Design review of the part built by this model. Coordinates are the model's own, in mm. A direction names the side the tool comes from. Round coordinates to 2 decimals unless told otherwise and drop trailing zeros. Order: outer loops, then holes, each group sorted by start corner. A loop starts at its lowest first (then second) coordinate and runs counter-clockwise, first axis right, second up.
from build123d import *

# Parameters (mm, degrees)
SKETCH1_W                       = 30
SKETCH1_H                       = 194.2
SKETCH1_H_2                     = 27
SKETCH1_H_3                     = 261.4
EXTRUDE1_DEPTH                  = 15
FILLET1_R                       = 10
EXTRUDE2_DEPTH                  = 10
SKETCH3_W                       = 80
SKETCH3_H                       = 25
EXTRUDE3_DEPTH                  = 30
SKETCH5_W                       = 70
SKETCH5_H                       = 20
EXTRUDE4_DEPTH                  = 24
FILLET2_R                       = 10
EXTRUDE5_REACH                  = 432.349
SKETCH6_R                       = 4.029178008
SKETCH7_W                       = 30
SKETCH7_H                       = 263.372286267
EXTRUDE6_DEPTH                  = 427.91910061
EXTRUDE7_DEPTH                  = 100
SKETCH9_W                       = 30
SKETCH9_H                       = 136.58118173
EXTRUDE8_DEPTH                  = 10
F_1_4_0_25_DIAMETER_HOLE1_D     = 6.35
F_1_4_0_25_DIAMETER_HOLE1_DEPTH = 10
F_1_4_0_25_DIAMETER_HOLE1_TIP   = 1.907732465
EXTRUDE12_DEPTH                 = 20
EXTRUDE12_DEPTH_BACK            = 30
SKETCH11_W                      = 15
SKETCH11_H                      = 6.378618897


with BuildPart() as part:
    # Sketch1 → Extrude1 (new body)
    with BuildSketch(Plane.XY):
        with Locations((15, 322.665015772)):
            Rectangle(SKETCH1_W, SKETCH1_H)
        with BuildLine():
            Line((30, 225.565015772), (30, 198.565015772))
            Line((30, 198.565015772), (50, 198.565015772))
            ThreePointArc((50, 198.565015772), (63.5, 212.065015772), (50, 225.565015772))
            Line((50, 225.565015772), (30, 225.565015772))
        make_face()
        with Locations((15, 212.065015772)):
            Rectangle(SKETCH1_W, SKETCH1_H_2)
        with BuildLine():
            Line((-20, 198.565015772), (0, 198.565015772))
            Line((0, 198.565015772), (0, 225.565015772))
            Line((0, 225.565015772), (-20, 225.565015772))
            ThreePointArc((-20, 225.565015772), (-33.5, 212.065015772), (-20, 198.565015772))
        make_face()
        with Locations((15, 67.865015772)):
            Rectangle(SKETCH1_W, SKETCH1_H_3)
    extrude(amount=EXTRUDE1_DEPTH)

    # Fillet1
    fillet1_edges = [part.edges().sort_by_distance(p)[0] for p in [
        (0, 419.765015772, 7.5),
        (30, 419.765015772, 7.5),
        (30, -62.834984228, 7.5),
        (0, -62.834984228, 7.5),
    ]]
    fillet(fillet1_edges, radius=FILLET1_R)

    # Sketch2 → Extrude2 (cut)
    with BuildSketch(Plane(origin=(0, 0, 0), x_dir=(-1, 0, 0), z_dir=(0, 0, -1))):
        with BuildLine():
            Line((-50, 225.565015772), (-30, 225.565015772))
            Line((-30, 225.565015772), (-30, 198.565015772))
            Line((-30, 198.565015772), (-50, 198.565015772))
            ThreePointArc((-50, 198.565015772), (-63.5, 212.065015772), (-50, 225.565015772))
        make_face()
        with BuildLine():
            Line((0, 198.565015772), (20, 198.565015772))
            ThreePointArc((20, 198.565015772), (33.5, 212.065015772), (20, 225.565015772))
            Line((20, 225.565015772), (0, 225.565015772))
            Line((0, 225.565015772), (0, 198.565015772))
        make_face()
    extrude(amount=-EXTRUDE2_DEPTH, mode=Mode.SUBTRACT)

    # Sketch3 → Extrude3 (add)
    with BuildSketch(Plane.XY.offset(15)):
        with Locations((15, 407.265015772)):
            Rectangle(SKETCH3_W, SKETCH3_H)
    extrude(amount=EXTRUDE3_DEPTH)

    # Sketch5 → Extrude4 (cut)
    with BuildSketch(Plane.XY.offset(45)):
        with Locations((15, 409.765015772)):
            Rectangle(SKETCH5_W, SKETCH5_H)
    extrude(amount=-EXTRUDE4_DEPTH, mode=Mode.SUBTRACT)

    # Fillet2
    fillet2_edges = [part.edges().sort_by_distance(p)[0] for p in [
        (52.5, 419.765015772, 45),
        (-22.5, 419.765015772, 45),
    ]]
    fillet(fillet2_edges, radius=FILLET2_R)

    # Sketch6 → Extrude5 (add, up to next)
    with BuildSketch(Plane.ZY.offset(-50), mode=Mode.PRIVATE) as extrude5_sk1:
        with Locations(Location((35, 413.847695375, 0), (0, 0, 180))):
            Circle(SKETCH6_R)
    extrude5_tool1 = extrude(extrude5_sk1.sketch, amount=EXTRUDE5_REACH, mode=Mode.PRIVATE) - part.part
    add(extrude5_tool1.solids().sort_by_distance((50, 413.847695, 35))[0])

    # Sketch7 → Extrude6 (cut, through all)
    with BuildSketch(Plane(origin=(0, 0, 0), x_dir=(-1, 0, 0), z_dir=(0, 0, -1))):
        with Locations((-15, 66.878872639)):
            Rectangle(SKETCH7_W, SKETCH7_H)
    extrude(amount=-EXTRUDE6_DEPTH, mode=Mode.SUBTRACT)

    # Sketch8 → Extrude7 (add)
    with BuildSketch(Plane(origin=(0, 0, 0), x_dir=(-1, 0, 0), z_dir=(0, 0, -1))):
        Polygon((-30, 198.565015772), (0, 198.565015772), (0, 225.565015772), (-5, 225.565015772), (-5, 203.565015772), (-25, 203.565015772), (-25, 225.565015772), (-30, 225.565015772), align=None)
    extrude(amount=EXTRUDE7_DEPTH)

    # Sketch9 → Extrude8 (add)
    with BuildSketch(Plane(origin=(0, 0, -100), x_dir=(-1, 0, 0), z_dir=(0, 0, -1))):
        with Locations((-15, 157.274424907)):
            Rectangle(SKETCH9_W, SKETCH9_H)
    extrude(amount=EXTRUDE8_DEPTH)

    # 1/4 (0.25) Diameter Hole1
    with Locations(Plane(origin=(-20, 212.065015772, 10), x_dir=(-1, 0, 0), z_dir=(0, 0, -1))):
        with Locations((0, 0), (-70, 0)):
            Hole(F_1_4_0_25_DIAMETER_HOLE1_D / 2, depth=F_1_4_0_25_DIAMETER_HOLE1_DEPTH)
            with Locations((0, 0, -(F_1_4_0_25_DIAMETER_HOLE1_DEPTH + F_1_4_0_25_DIAMETER_HOLE1_TIP / 2))):  # 118° drill point
                Cone(0, F_1_4_0_25_DIAMETER_HOLE1_D / 2, F_1_4_0_25_DIAMETER_HOLE1_TIP, mode=Mode.SUBTRACT)

    # Sketch11 → Extrude12 (add, two sides: drawn at the far end of the back side and taken through both)
    with BuildSketch(Plane.XZ.offset(-88.983834042).offset(-EXTRUDE12_DEPTH_BACK)):
        Polygon((0, -116.378618897), (-22.784065685, -134.102681991), (-22.784065685, -127.724063095), (0, -110), align=None)
        with Locations((22.5, -113.189309449)):
            Rectangle(SKETCH11_W, SKETCH11_H)
        with Locations((7.5, -113.189309449)):
            Rectangle(SKETCH11_W, SKETCH11_H)
        Polygon((30, -116.378618897), (52.784065685, -134.102681991), (52.784065685, -127.724063095), (30, -110), align=None)
    extrude(amount=EXTRUDE12_DEPTH + EXTRUDE12_DEPTH_BACK)


solid = part.part
1) Take a section at C-C on y = 160. Give the boundary of the cut face in (x, z), plus the area to 3 significant figures.
Results:
outline: (0, -110) - (30, -110) - (30, -100) - (0, -100) - close
area: 300 mm2
2) The part is to be moulded in two halves that separate along X. For faces 1 (the face through (27.148, 416.758, 7.605)), 2 (the face through (15, 173, -110)), 3 (the face through (15, 399.765, 33)), say which applies: released by +X, released by -X, zero draft, split by the parting line, or undercut.
Results:
face 1: released by +X
face 2: zero draft
face 3: undercut
3) Take a section at A-A on x = -10.5. Give the boundary of the cut face in (y, z), plus the area to 3 significant figures.
Results:
outline: (68.98, -124.55) - (118.98, -124.55) - (118.98, -118.17) - (68.98, -118.17) - close; (198.57, 10) - (225.57, 10) - (225.57, 15) - (198.57, 15) - close; (394.77, 15) - (419.77, 15) - (419.77, 21) - (399.77, 21) - (399.77, 45) - (394.77, 45) - close; circle Ø8.06 at (413.85, 35)
area: 775 mm2
4) Take a section at D-D on y = 293.5. Give the boundary of the cut face in (x, z), plus the area to 3 significant figures.
Results:
outline: (0, 0) - (30, 0) - (30, 15) - (0, 15) - close
area: 450 mm2
5) To check wall thickness, follow line 1 along Z through (x, y) = (10.5, 368.5); line 2 along Y through (x, z) = (50, 13); line 3 along Z through (x, y) = (26.5, 214). State the ranges of each line that lie inside material, in increasing order.
Results:
line 1: z = 0 to 15
line 2: y = 198.57 to 208.89, 215.24 to 225.57
line 3: z = -110 to 15
6) Take a section at B-B on z = -33. Give the boundary of the cut face in (x, y), plus the area to 3 significant figures.
Results:
outline: (0, 198.57) - (30, 198.57) - (30, 225.57) - (25, 225.57) - (25, 203.57) - (5, 203.57) - (5, 225.57) - (0, 225.57) - close
area: 370 mm2
7) Clearance check with flat-ended pins moving along their axes: P1, Ø21.5, axis at x = -8.5, y = 215.5, coming from the -Z side; P2, Ø3, axis at x = 10, z = -103.5, coming from the -Y side; P3, Ø5, axis at y = 97.5, z = -130, coming from the -X side. State where each tip first meets the part, or that it passes through.
Results:
P1: stops at z = -110
P2: stops at y = 88.98
P3: stops at x = -22.78
8) For faces 4 (the face through (46.5, 212.3, 10)), 5 (the face through (-16.5, 212.3, 10)), 6 (the face through (15, 198.565, -38)), 7 (the face through (5, 215, -49)), list the 3-axis set-ups (+Z, -Z, +X, -X, +Y, -Y) from which the entire face can be reached by the end or side of a thin tool; tool diameter is ignored.
Results:
face 4: -Z, +X, +Y, -Y
face 5: -Z, -X, +Y, -Y
face 6: +Z, +X, -X, -Y
face 7: +Y
